Input: part model. Units: mm. Frame: model coordinates. A direction names the side the tool comes from. Give positions to 0.01 mm unless a question says otherwise; leave off trailing zeros. Loops run counter-clockwise (first coordinate to the right, second up) from the corner with the lowest first, then second, coordinate; pieces in that order, holes last. Notation, with made-up numbers: (-18.5, 31) - (-8.5, 31) arc R35 ccw to (-8.5, 65) - close; hole circle Ø8 at (-7.5, 4). An arc over 180 degrees is marked (long way). Answer as a JSON object with one key per item and string values. Group by question number.
(1) Section query B-B (y = 16). Return loops of the section in (x, z).
(2) Section query A-A (x = 0). Return loops of the section in (y, z).
(3) Access query for faces 1 (the cylindrical face through (-1.214, 6.945, 1.578)), 2 (the flat face through (-7, 3, 0)), 3 (the flat face through (-1.6, -8.4, 1.5)). Directions: +Z, -Z, +X, -X, +Y, -Y. A direction counts if a zero-diameter tool reaches every point of the face in a straight line with its end or side. Return the directions, or none.
(4) Pin query (flat end, axial travel): P1, Ø1, axis at x = -8, z = 1.5, coming from the -Y side; P2, Ø0.6, axis at x = 4.5, y = -7.5, coming from the -Z side; P3, Ø1, axis at y = 9, z = 2, coming from the +X side. Return the tip coordinate at first contact, or that it passes through.
(5) Section query D-D (x = 12.5). Return loops of the section in (y, z).
(6) Section query C-C (z = 1.05). Count the separate pieces of the cut face and the enclosed holes in it, plus the area to 3 significant figures.
(7) Mould query, pull axis X, two halves, no side actions, for faces 4 (the flat face through (-3.9, 6.6, 0)), 5 (the flat face through (0.5, -9, 2)), 6 (the cylindrical face through (0, 19.5, 1.6)). Classes: +X half, -X half, draft (parallel to the pull), parting line (faces both ways), or undercut.
(8) Material intervals for L1, parallel to Y at x = 0, z = 1.1; L2, parallel to Y at x = 10.5, z = 0.9; L3, parallel to Y at x = 6, z = 2.35, sorted ascending.
```python
from build123d import *

# Parameters (mm, degrees)
SKETCH_1_R               = 7.05
EXTRUDE_1_DEPTH          = 3.2
SKETCH_2_R               = 1.6
CUT_EXTRUDE_1_DEPTH      = 10
CUT_EXTRUDE_START        = 27.729945754
CUT_EXTRUDE_3_DEPTH      = 31.729945754
PATTERN_CIRCULAR_1_COUNT = 18
SKETCH_4_R               = 9.1
SKETCH_4_R_2             = 8.1
CUT_EXTRUDE_4_DEPTH      = 1.5


with BuildPart() as part:
    # 草图1 → 凸台-拉伸1 (new body)
    with BuildSketch(Plane.XY):
        with BuildLine():
            ThreePointArc((-14.058374697, -11.241089844), (0, -18), (14.058374697, -11.241089844))
            ThreePointArc((14.058374697, -11.241089844), (16.887495374, -9.75), (16.76425672, -6.554364701))
            ThreePointArc((16.76425672, -6.554364701), (15.588457268, 9), (2.705882023, 17.795454545))
            ThreePointArc((2.705882023, 17.795454545), (0, 19.5), (-2.705882023, 17.795454545))
            ThreePointArc((-2.705882023, 17.795454545), (-15.588457268, 9), (-16.76425672, -6.554364701))
            ThreePointArc((-16.76425672, -6.554364701), (-16.887495374, -9.75), (-14.058374697, -11.241089844))
        make_face()
        Circle(SKETCH_1_R, mode=Mode.SUBTRACT)
    extrude(amount=EXTRUDE_1_DEPTH)

    # 草图2 → 切除-拉伸1 (cut)
    with BuildSketch(Plane.XY.offset(3.2)):
        with Locations((0, 17)):
            Circle(SKETCH_2_R)
        with Locations((14.722431864, -8.5)):
            Circle(SKETCH_2_R)
        with Locations((-14.722431864, -8.5)):
            Circle(SKETCH_2_R)
    extrude(amount=-CUT_EXTRUDE_1_DEPTH, mode=Mode.SUBTRACT)

    # 草图3 → 切除-拉伸3 (cut)
    with BuildSketch(Plane(origin=(0, 0, 0), x_dir=(-1, 0, 0), z_dir=(0, 0, -1)).offset(CUT_EXTRUDE_START)):
        with BuildLine():
            ThreePointArc((-0.5, 7.032247152), (0, 7.05), (0.5, 7.032247152))
            Line((0.5, 7.032247152), (0.5, 11))
            Line((0.5, 11), (-0.5, 11))
            Line((-0.5, 11), (-0.5, 7.032247152))
        make_face()
    cut_extrude_3 = extrude(amount=-CUT_EXTRUDE_3_DEPTH, mode=Mode.SUBTRACT)

    # 阵列(圆周)1: 切除-拉伸3 ×18 about axis
    pattern_circular_1_axis = Axis((0, 0, 0), (0, 0, 1))
    for i in range(1, PATTERN_CIRCULAR_1_COUNT):
        add(cut_extrude_3.rotate(pattern_circular_1_axis, i * 360 / PATTERN_CIRCULAR_1_COUNT), mode=Mode.SUBTRACT)

    # 草图4 → 切除-拉伸4 (cut)
    with BuildSketch(Plane(origin=(0, 0, 0), x_dir=(-1, 0, 0), z_dir=(0, 0, -1))):
        Circle(SKETCH_4_R)
        Circle(SKETCH_4_R_2, mode=Mode.SUBTRACT)
    extrude(amount=-CUT_EXTRUDE_4_DEPTH, mode=Mode.SUBTRACT)


solid = part.part
```
Recorded:
{
 "1": {"outline": "(-8.25, 0) - (-1.25, 0) - (-1.25, 3.2) - (-8.25, 3.2) - close; (1.25, 0) - (8.25, 0) - (8.25, 3.2) - (1.25, 3.2) - close"},
 "2": {"outline": "(-18, 0) - (-11, 0) - (-11, 3.2) - (-18, 3.2) - close; (11, 0) - (15.4, 0) - (15.4, 3.2) - (11, 3.2) - close; (18.6, 0) - (19.5, 0) - (19.5, 3.2) - (18.6, 3.2) - close"},
 "3": {"face 1": "+Z, -Z", "face 2": "-Z, +X, -X, +Y, -Y", "face 3": "-Z"},
 "4": {"P1": "stops at y = -16.36", "P2": "stops at z = 1.5", "P3": "stops at x = 15.87"},
 "5": {"outline": "(-12.95, 0) - (12.95, 0) - (12.95, 3.2) - (-12.95, 3.2) - close"},
 "6": {"separate pieces": "19", "enclosed holes": "4", "area": "748 mm^2"},
 "7": {"face 4": "draft", "face 5": "undercut", "face 6": "parting line"},
 "8": {"L1": "y = -18 to -11, 11 to 15.4, 18.6 to 19.5", "L2": "y = -14.62 to -2.36, -1.34 to 1.34, 2.36 to 14.62", "L3": "y = -16.97 to -7.93, -6.37 to -4.04, 4.04 to 6.37, 7.93 to 16.97"}
}
